```python
from build123d import *

# Parameters (mm, degrees)
F0_W     = 175
F0_H     = 130
F0_R     = 7.5
F1_DEPTH = 25.4


with BuildPart() as f1:
    # F0 (on Top) → F1 (new body)
    with BuildSketch(Plane.XY):
        with Locations((-0.0971, 0.811385)):
            Rectangle(F0_W, F0_H)
        with Locations((-65.0971, -53.288615)):
            Circle(F0_R, mode=Mode.SUBTRACT)
        with Locations((-39.6971, -53.288615)):
            Circle(F0_R, mode=Mode.SUBTRACT)
        with Locations((-14.2971, -53.288615)):
            Circle(F0_R, mode=Mode.SUBTRACT)
        with Locations((-65.0971, -27.888615)):
            Circle(F0_R, mode=Mode.SUBTRACT)
        with Locations((-65.0971, -2.488615)):
            Circle(F0_R, mode=Mode.SUBTRACT)
        with Locations((-39.6971, -27.888615)):
            Circle(F0_R, mode=Mode.SUBTRACT)
        with Locations((-14.2971, -27.888615)):
            Circle(F0_R, mode=Mode.SUBTRACT)
        with Locations((-39.6971, -2.488615)):
            Circle(F0_R, mode=Mode.SUBTRACT)
        with Locations((-14.2971, -2.488615)):
            Circle(F0_R, mode=Mode.SUBTRACT)
        with Locations((11.1029, -53.288615)):
            Circle(F0_R, mode=Mode.SUBTRACT)
        with Locations((36.5029, -53.288615)):
            Circle(F0_R, mode=Mode.SUBTRACT)
        with Locations((61.9029, -53.288615)):
            Circle(F0_R, mode=Mode.SUBTRACT)
        with Locations((11.1029, -27.888615)):
            Circle(F0_R, mode=Mode.SUBTRACT)
        with Locations((36.5029, -27.888615)):
            Circle(F0_R, mode=Mode.SUBTRACT)
        with Locations((11.1029, -2.488615)):
            Circle(F0_R, mode=Mode.SUBTRACT)
        with Locations((36.5029, -2.488615)):
            Circle(F0_R, mode=Mode.SUBTRACT)
        with Locations((61.9029, -27.888615)):
            Circle(F0_R, mode=Mode.SUBTRACT)
        with Locations((61.9029, -2.488615)):
            Circle(F0_R, mode=Mode.SUBTRACT)
        with Locations((-65.0971, 22.911385)):
            Circle(F0_R, mode=Mode.SUBTRACT)
        with Locations((-39.6971, 22.911385)):
            Circle(F0_R, mode=Mode.SUBTRACT)
        with Locations((-14.2971, 22.911385)):
            Circle(F0_R, mode=Mode.SUBTRACT)
        with Locations((-65.0971, 48.311385)):
            Circle(F0_R, mode=Mode.SUBTRACT)
        with Locations((-39.6971, 48.311385)):
            Circle(F0_R, mode=Mode.SUBTRACT)
        with Locations((-14.2971, 48.311385)):
            Circle(F0_R, mode=Mode.SUBTRACT)
        with Locations((11.1029, 22.911385)):
            Circle(F0_R, mode=Mode.SUBTRACT)
        with Locations((36.5029, 22.911385)):
            Circle(F0_R, mode=Mode.SUBTRACT)
        with Locations((61.9029, 22.911385)):
            Circle(F0_R, mode=Mode.SUBTRACT)
        with Locations((11.1029, 48.311385)):
            Circle(F0_R, mode=Mode.SUBTRACT)
        with Locations((36.5029, 48.311385)):
            Circle(F0_R, mode=Mode.SUBTRACT)
        with Locations((61.9029, 48.311385)):
            Circle(F0_R, mode=Mode.SUBTRACT)
    extrude(amount=F1_DEPTH)


solid = f1.part
```
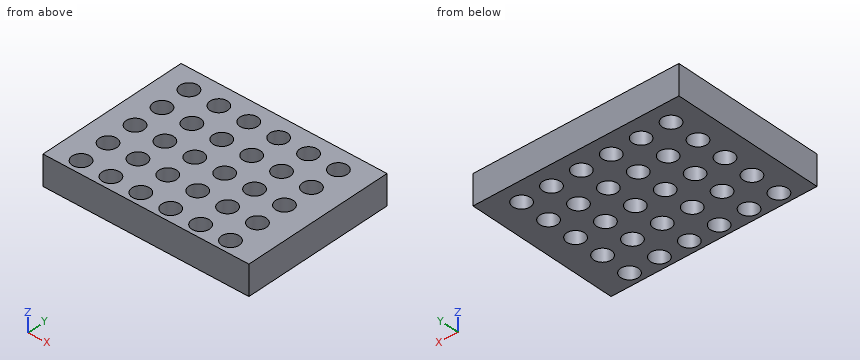
Geometry check sheet. Reference: the model listing, model coordinates, mm. Round coordinates to 2 decimals unless told otherwise and drop trailing zeros. Order: outer loops, then holes, each group sorted by start corner. A loop starts at its lowest first (then second) coordinate and runs counter-clockwise, first axis right, second up. Notation, with made-up numbers: (57.25, 44.5) - (86.25, 44.5) arc R13 ccw to (86.25, 61.5) - close; hole circle Ø11 at (-3.75, 5). An arc over 180 degrees is marked (long way). Use a Markdown table: item, result. Add a question column.
1) Gauge pin test, flat end, axial feed: P1, Ø9, axis at x = -39.7, y = -2.49, coming from the +Z side. Record the tip position at first contact, or that the pin passes through.
2) Section check D-D (x = 37). Record the cut outline in (y, z), then the cut area to 3 significant figures.
3) Section check C-C (z = 3.25). Count the separate pieces of the cut face and the enclosed holes in it, then the cut area to 3 significant figures.
4) Section check A-A (y = -22.5). Record the cut outline in (x, z), then the cut area to 3 significant figures.
5) Thickness scan on line 1 along Y through (x, z) = (-40.5, 24.25); line 2 along Y through (x, z) = (12.5, 8.5). Record the ranges inside material, lowest first.
6) Section check B-B (x = -43.5). Record the cut outline in (y, z), then the cut area to 3 significant figures.
Established:
| question | item | result |
|---|---|---|
| 1 | P1 | through |
| 2 | outline | (-64.19, 0) - (-60.77, 0) - (-60.77, 25.4) - (-64.19, 25.4) - close; (-45.81, 0) - (-35.37, 0) - (-35.37, 25.4) - (-45.81, 25.4) - close; (-20.41, 0) - (-9.97, 0) - (-9.97, 25.4) - (-20.41, 25.4) - close; (4.99, 0) - (15.43, 0) - (15.43, 25.4) - (4.99, 25.4) - close; (30.39, 0) - (40.83, 0) - (40.83, 25.4) - (30.39, 25.4) - close; (55.79, 0) - (65.81, 0) - (65.81, 25.4) - (55.79, 25.4) - close |
| 2 | area | 1,400 mm2 |
| 3 | separate pieces | 1 |
| 3 | enclosed holes | 30 |
| 3 | area | 17,400 mm2 |
| 4 | outline | (-87.6, 0) - (-70.31, 0) - (-70.31, 25.4) - (-87.6, 25.4) - close; (-59.88, 0) - (-44.91, 0) - (-44.91, 25.4) - (-59.88, 25.4) - close; (-34.48, 0) - (-19.51, 0) - (-19.51, 25.4) - (-34.48, 25.4) - close; (-9.08, 0) - (5.89, 0) - (5.89, 25.4) - (-9.08, 25.4) - close; (16.32, 0) - (31.29, 0) - (31.29, 25.4) - (16.32, 25.4) - close; (41.72, 0) - (56.69, 0) - (56.69, 25.4) - (41.72, 25.4) - close; (67.12, 0) - (87.4, 0) - (87.4, 25.4) - (67.12, 25.4) - close |
| 4 | area | 2,850 mm2 |
| 5 | line 1 | -64.19 to -60.75, -45.83 to -35.35, -20.43 to -9.95, 4.97 to 15.45, 30.37 to 40.85, 55.77 to 65.81 |
| 5 | line 2 | -64.19 to -60.66, -45.92 to -35.26, -20.52 to -9.86, 4.88 to 15.54, 30.28 to 40.94, 55.68 to 65.81 |
| 6 | outline | (-64.19, 0) - (-59.75, 0) - (-59.75, 25.4) - (-64.19, 25.4) - close; (-46.82, 0) - (-34.35, 0) - (-34.35, 25.4) - (-46.82, 25.4) - close; (-21.42, 0) - (-8.95, 0) - (-8.95, 25.4) - (-21.42, 25.4) - close; (3.98, 0) - (16.45, 0) - (16.45, 25.4) - (3.98, 25.4) - close; (29.38, 0) - (41.85, 0) - (41.85, 25.4) - (29.38, 25.4) - close; (54.78, 0) - (65.81, 0) - (65.81, 25.4) - (54.78, 25.4) - close |
| 6 | area | 1,660 mm2 |
